Design review of the part shown in the three views and the two pictorial views. Dimensions are in mm from the part's minimum x, y and z. Coordinates: 2 decimals unless noted, no trailing zeros. Write each loop counter-clockwise with the first axis right and the second up, starting at its lowest first coordinate (ties: lowest second). Pieces come first, ordered by that corner, then holes. Notation, with made-up numbers: (38.5, 41) -> (97.5, 41) arc R25 ccw to (97.5, 59) -> close; hole circle Ø11 at (57.5, -3.5). An arc over 180 degrees is marked (long way). Write each question's results on one line, items separated by ' | '.
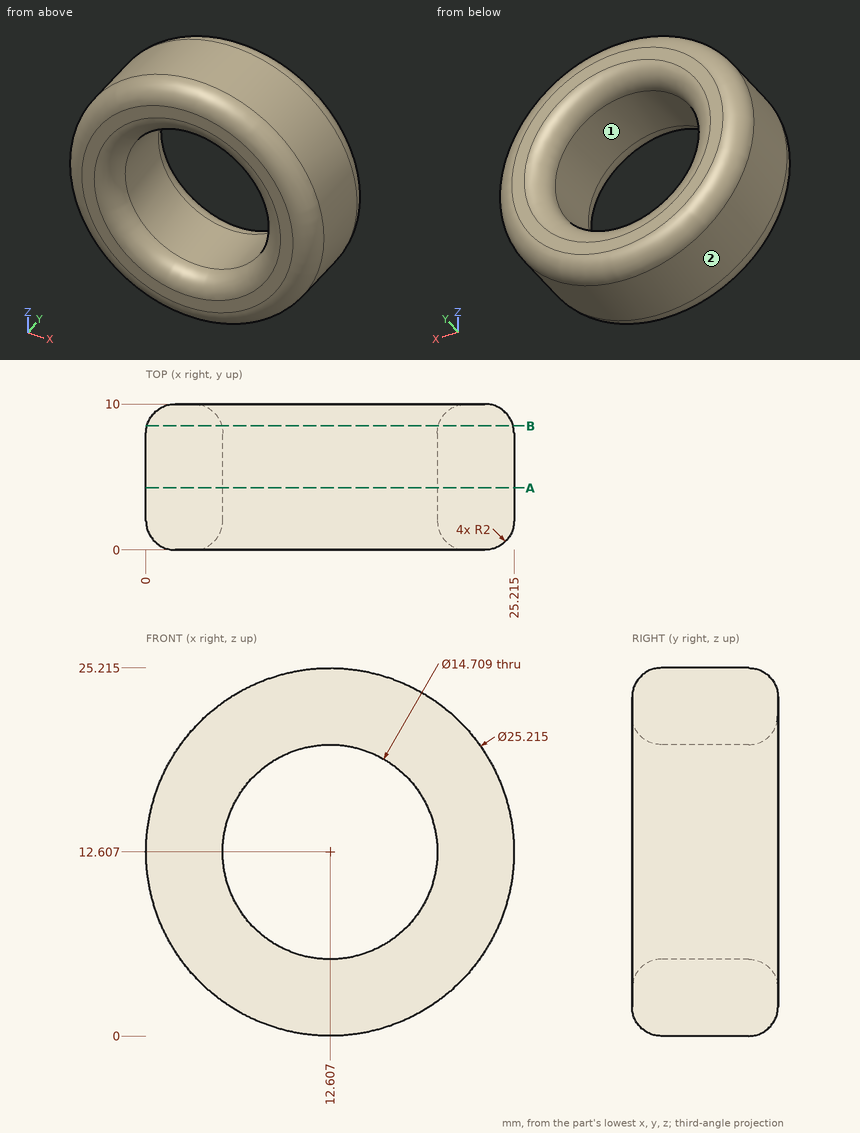
Q1. Add section B-B (y = 8.5). Write out the cut boundary in (x, z) (1 decimal).
Solution:
outline: circle Ø25.1 at (12.6, 12.6); hole circle Ø14.8 at (12.6, 12.6)
Q2. For line 1 (Z direction, x = 12.5, y = 4.5) (1 decimal); line 2 (Y direction, x = 9, z = 2.5); line 3 (X direction, y = 3.5, z = 9) (1 decimal), list the stretches that pass through material, from the lowest coordinate up. Write a range as from..to.
Solution:
line 1: 0..5.3, 20..25.2 | line 2: 0..10 | line 3: 0.5..6.2, 19..24.7
Q3. Add section A-A (y = 4.25). Write out the cut boundary in (x, z) (1 decimal).
Solution:
outline: circle Ø25.2 at (12.6, 12.6); hole circle Ø14.7 at (12.6, 12.6)
Q4. Clearance check with flat-ended pins moving along their axes: P1, Ø1, axis at x = 6.5, z = 5.5, coming from the -Y side; P2, Ø5, axis at y = 3.5, z = 7, coming from the -X side; P3, Ø6, axis at x = 2.5, y = 8.5, coming from the +Z side. State where each tip first meets the part, or that it passes through.
Solution:
P1: y = 0 | P2: x = 0.39 | P3: z = 23
Q5. Draft analysis for pull direction X (two halves, no side actions). For the marked faces 1 and 2, state which applies: pulls with the +X half, pulls with the -X half, needs draft (parallel to the pull), parting line crosses it, or undercut.
Solution:
face 1: undercut | face 2: parting line crosses it
